CAD build for the part. Positions are in the model's coordinates, mm. A direction names the side the tool comes from. Round coordinates to 2 decimals unless told otherwise and drop trailing zeros. Write each loop counter-clockwise with the first axis right and the second up, starting at its lowest first coordinate (ties: lowest second). Pieces come first, ordered by that corner, then holes. Notation, with made-up numbers: (38.25, 76) - (91.25, 76) arc R24 cw to (91.25, 91) - close; hole circle Ø11 at (9, 63.25). An arc over 180 degrees is marked (long way). Put each result on its own line as item: value. Start each with the question number.
Item 1: Drill centre lines: line 1 (X direction, y = -28.45, z = -4.1); line 2 (Y direction, x = 19, z = 6); line 3 (X direction, y = -6, z = -2.25). Where is each one in solid material? Low to high. Write a range as from..to.
Item 2: 3-axis set-ups, long thin cutter, end or side, ignore diameter. For faces 1 (the flat face through (7.7, -2, -2)), 2 (the cylindrical face through (10.62, -1.57, 8.21)), 3 (the cylindrical face through (4.155, -28.014, 8.396)): which of +Z, -Z, +X, -X, +Y, -Y reach the whole face in a straight line?
Item 3: Cut at A-A (y = 2). Give the cut face in (x, z).
Item 4: Pin check, flat tips, straight feed: pin 1 Ø0.6 at (y, z) = (-25, 9.5) entering from +X; pin 2 Ø2.5 at (x, y) = (20, 0.5) entering from -Z; pin 3 Ø3 at (x, y) = (13.02, -1.67) entering from -Z. Stop position of each tip, or through.
Item 5: Mould opens along X. For faces 4 (the flat face through (0, -2, -2)), 5 (the cylindrical face through (3.5, -17.97, 10.18)), 6 (the flat face through (18, 6.05, 5)) say: released by +X, released by -X, zero draft, split by the parting line, or undercut.
Autodesk Inventor part; units mm, degrees
ref_plane "YZ Plane" through (0, 0, 0) normal (1, 0, 0) x (0, 1, 0)
ref_plane "XZ Plane" through (0, 0, 0) normal (0, 1, 0) x (-1, 0, 0)
ref_plane "XY Plane" through (0, 0, 0) normal (0, 0, 1) x (1, 0, 0)
ref_plane "Work Plane1" through (3.85, 70.2125, 8.85) normal (1, 0, 0) x (0, 0, 1)
sketch "Sketch1" plane through (3.85, 70.2125, 8.85) normal (1, 0, 0) x (0, 0, 1)
  line L0 (-8.85, 70.2125) -> (-17.05, 70.2125) construction
  line L1 (-17.05, 70.2125) -> (-17.05, 65.2125) construction
  line L2 (-8.85, 65.2125) -> (-17.05, 65.2125) construction
  line L3 (-8.85, 70.2125) -> (-8.85, 65.2125) construction
  arc A0 (-25.45, 97.2125) -> (-0.45, 97.2125) centre (-12.95, 114.7438) ccw construction
  arc A1 (-0.45, 99.2125) -> (-25.45, 99.2125) centre (-12.95, 81.6813) ccw construction
  line L4 (-0.45, 99.2125) -> (-0.45, 97.2125) construction
  line L5 (-25.45, 99.2125) -> (-25.45, 97.2125) construction
  line L6 (-12.95, -45.926) -> (-12.95, 188.756) construction
  line L7 (-10.1686, 64.1631) -> (-10.1686, 77.6475)
  line L8 (-10.1686, 77.6475) -> (-3.1244, 95.5852)
  line L9 (-3.1244, 100.8399) -> (-3.1244, 103.9225)
  line L10 (-3.1244, 103.9225) -> (1.3329, 103.9225)
  line L11 (1.3329, 103.9225) -> (1.3329, 64.1631)
  line L12 (1.3329, 64.1631) -> (-10.1686, 64.1631)
  arc A2 (-3.1244, 95.5852) -> (-0.45, 97.2125) centre (-12.95, 114.7438) ccw
  arc A3 (-0.45, 99.2125) -> (-3.1244, 100.8399) centre (-12.95, 81.6813) ccw
  line L13 (-0.45, 97.2125) -> (-0.45, 99.2125)
revolve "Revolution1" add sketch "Sketch1" angle 200 mid plane about axis through (3.85, 116.1385, -4.1) along (0, -1, 0)
sketch "Sketch2" plane through (3.85, 6.0495, -4.1) normal (0, 1, 0) x (1, 0, 0)
  circle A0 centre (0, 0) radius 2.8472
  line L0 (-3.85, -4.1) -> (3.85, -4.1)
  line L1 (3.85, -4.1) -> (3.85, 4.1)
  line L2 (3.85, 4.1) -> (-3.85, 4.1)
  line L3 (-3.85, 4.1) -> (-3.85, -4.1)
  line L4 (-3.55, -3.8) -> (3.55, -3.8)
  line L5 (3.55, -3.8) -> (3.55, 3.8)
  line L6 (3.55, 3.8) -> (-3.55, 3.8)
  line L7 (-3.55, 3.8) -> (-3.55, -3.8)
  dimension "d1" = 0.3
extrude "Extrusion1" cut sketch "Sketch2" against normal through all contours A0 | L3 L2 L1 L0 | L7 L6 L5 L4
sketch "Sketch3" plane through (3.85, 6.0495, -4.1) normal (0, 1, 0) x (1, 0, 0)
  arc A0 (-14.0659, 2.4802) -> (14.0659, 2.4802) centre (0, 0) ccw
  line L0 (-14.2797, -0.3038) -> (-14.2797, -14.2829)
  line L1 (-14.2797, -0.3038) -> (-0.3006, -0.3038) construction
  line L2 (-14.2797, -14.2829) -> (0, -14.2829)
  line L3 (14.2797, -0.3038) -> (14.2797, -14.2829)
  line L4 (14.2797, -14.2829) -> (0, -14.2829)
  line L5 (14.2797, -14.2829) -> (17.2797, -14.2829)
  line L6 (17.2797, -14.2829) -> (17.2797, 0)
  line L7 (17.2797, 0) -> (14.2797, 0)
  line L8 (14.2797, 0) -> (14.2797, -14.2829)
  point P0 (-3.85, -4.1)
  dimension "d4" = 90
  dimension "d11" = 3
extrude "Extrusion2" add sketch "Sketch3" against normal blind 12
sketch "Sketch6" plane through (-10.4297, 6.0495, 10.1829) normal (0, 0, 1) x (1, 0, 0)
  line L0 (13.7983, -35.2418) -> (21.7983, -35.2418)
  line L1 (21.7983, -35.2418) -> (21.7983, -27.2418)
  line L2 (21.7983, -27.2418) -> (13.7983, -27.2418)
  line L3 (13.7983, -27.2418) -> (13.7983, -35.2418)
  line L4 (13.7983, -35.2418) -> (21.7983, -27.2418)
  line L5 (21.7983, -35.2418) -> (13.7983, -27.2418)
  circle A0 centre (13.4583, -31.2418) radius 1.4
  point P0 (10.4297, -6.0495)
  point P1 (17.7983, -31.2418)
  dimension "d12" = 8
  dimension "d13" = 8
extrude "Extrusion3" add sketch "Sketch6" against normal up to surface
sketch "Sketch7" plane through (-10.4297, 6.0495, 10.1829) normal (0, 0, 1) x (1, 0, 0)
  circle A0 centre (23.447, -7.7206) radius 1.4 construction
  circle A1 centre (2.8893, -7.9757) radius 1.4 construction
  circle A2 centre (13.4583, -31.2418) radius 1.4 construction
  circle A3 centre (13.4583, -31.2418) radius 2.4
  circle A4 centre (23.447, -7.7206) radius 2.4
  circle A5 centre (2.8893, -7.9757) radius 2.4
  point P0 (10.4297, -6.0495)
  dimension "d16" = 4.8
  dimension "d17" = 4.8
  dimension "d18" = 4.8
extrude "Extrusion4" cut sketch "Sketch7" against normal blind 4
properties part number "30_CUBE_OpenSIM_Beamexpander_v2"
Output values:
1. line 1: -10.43..-8.65, 16.35..18.13
1. line 2: -5.95..6.05
1. line 3: -10.31..0, 7.7..18.01
2. face 1: -Z, +Y, -Y
2. face 2: +Z
2. face 3: none
3. outline: (-10.43, -3.8) arc R14.28 ccw to (-10.22, -6.58) - (0, -4.78) - (0, 0) - (7.7, 0) - (7.7, -4.78) - (17.92, -6.58) arc R14.28 ccw to (18.13, -4.1) - (21.13, -4.1) - (21.13, 10.18) - (-10.43, 10.18) - close
4. pin 1: x = 11.37
4. pin 2: z = -4.1
4. pin 3: z = -5.98
5. face 4: undercut
5. face 5: split by the parting line
5. face 6: zero draft
